Verification items for the finished model (mm, model axes). Face numbers are marked on the shaded views. A direction names the side the tool comes from. Coordinates: 2 decimals unless noted, no trailing zeros. Order: outer loops, then holes, each group sorted by start corner. A loop starts at its lowest first (then second) coordinate and runs counter-clockwise, first axis right, second up. Notation, with made-up numbers: (88, 8) - (99, 8) arc R17 cw to (99, 37) - close; hole circle Ø11 at (31, 84). An arc over 180 degrees is marked (long way). Answer as CSV lines item,"result". Start each with the question number.
1. Go/stop test with flat-tipped pins: pin 1 (1.5 mm diameter, centred on y = 45.5, z = 10, fed in from -X); pin 2 (4 mm diameter, centred on y = 118, z = -8, fed in from -X); pin 3 (8 mm diameter, centred on x = -62, y = -13, fed in from +Z); pin 4 (8 mm diameter, centred on x = -92, z = -17, fed in from +Y). Record where each tip stops, or that it passes through.
2. Section check A-A (z = 4). Record the cut outline in (x, y).
3. Section check D-D (y = 135). Record the cut outline in (x, z), and give its area (3 significant figures).
4. Section check C-C (x = 0). Record the cut outline in (y, z), and give its area (3 significant figures).
5. Set-up check for the marked faces 1, 2 and 3: record each of +Z, -Z, +X, -X, +Y, -Y from which the full face is reachable in a straight line by a thin tool's end or side.
6. Section check B-B (y = -63.5). Record the cut outline in (x, z), and give its area (3 significant figures).
7. Material ranges on L1, parallel to X at y = -41.5, z = 2; L2, parallel to X at y = -66, z = -9.5; L3, parallel to Z at x = 100, y = -31.5, recorded low to high. Write a range as [from, to].
8. Mould release check, pull along X, two halves, no side actions. Record for the marked faces 4, 5 and 6: pulls with the +X half, pulls with the -X half, needs draft (parallel to the pull), parting line crosses it, or undercut.
from build123d import *

# Parameters (mm, degrees)
SKETCH1_R           = 50
BOSS_EXTRUDE1_DEPTH = 25
BOSS_EXTRUDE2_DEPTH = 10
SKETCH3_R           = 5
BOSS_EXTRUDE3_DEPTH = 1


with BuildPart() as part:
    # Sketch1 → Boss-Extrude1 (new body, symmetric)
    with BuildSketch(Plane.XY):
        Circle(SKETCH1_R)
    extrude(amount=BOSS_EXTRUDE1_DEPTH, both=True)

    # Sketch2 → Boss-Extrude2 (add, symmetric)
    with BuildSketch(Plane.XY):
        with BuildLine():
            Line((-21.510823847, 45.13628759), (-38.875641614, 143.617062891))
            ThreePointArc((-38.875641614, 143.617062891), (0, 153.617062891), (38.875641614, 143.617062891))
            Line((38.875641614, 143.617062891), (21.510823847, 45.13628759))
            ThreePointArc((21.510823847, 45.13628759), (0, 50), (-21.510823847, 45.13628759))
        make_face()
        with BuildLine():
            Line((104.938204074, -105.475824672), (28.333759762, -41.197063703))
            ThreePointArc((28.333759762, -41.197063703), (43.301270189, -25), (49.844583609, -3.939223887))
            Line((49.844583609, -3.939223887), (143.813845688, -38.14123822))
            ThreePointArc((143.813845688, -38.14123822), (133.036278919, -76.808531446), (104.938204074, -105.475824672))
        make_face()
        with BuildLine():
            Line((-143.813845688, -38.14123822), (-49.844583609, -3.939223887))
            ThreePointArc((-49.844583609, -3.939223887), (-43.301270189, -25), (-28.333759762, -41.197063703))
            Line((-28.333759762, -41.197063703), (-104.938204074, -105.475824672))
            ThreePointArc((-104.938204074, -105.475824672), (-133.036278919, -76.808531446), (-143.813845688, -38.14123822))
        make_face()
    extrude(amount=BOSS_EXTRUDE2_DEPTH, both=True)

    # Sketch3 → Boss-Extrude3 (add, symmetric)
    with BuildSketch(Plane.XY.offset(10)):
        with Locations((0, 135)):
            Circle(SKETCH3_R)
    extrude(amount=BOSS_EXTRUDE3_DEPTH, both=True)


solid = part.part
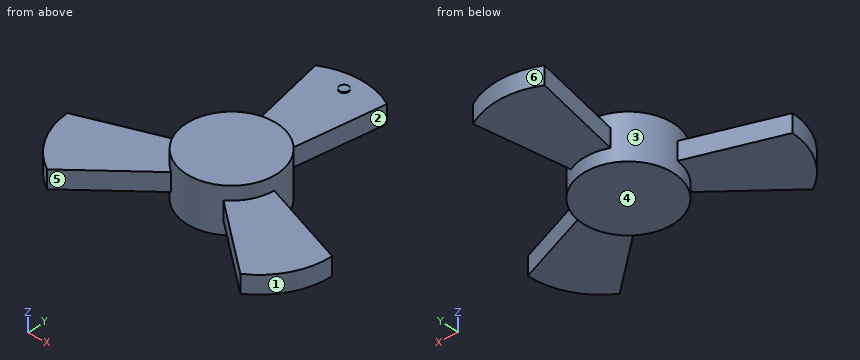
Evaluation:
1,pin 1,"stops at x = -22.3"
1,pin 2,"stops at x = -34.71"
1,pin 3,"stops at z = 10"
1,pin 4,"passes through"
2,outline,"(-143.81, -38.14) arc R80.57 ccw to (-104.94, -105.48) - (-28.33, -41.2) arc R50 ccw to (28.33, -41.2) - (104.94, -105.48) arc R80.57 ccw to (143.81, -38.14) - (49.84, -3.94) arc R50 ccw to (21.51, 45.14) - (38.88, 143.62) arc R80.57 ccw to (-38.88, 143.62) - (-21.51, 45.14) arc R50 ccw to (-49.84, -3.94) - close"
3,outline,"(-37.36, -10) - (37.36, -10) - (37.36, 10) - (5, 10) - (5, 11) - (-5, 11) - (-5, 10) - (-37.36, 10) - close"
3,area,"1,500 mm²"
4,outline,"(-50, -25) - (50, -25) - (50, -10) - (153.62, -10) - (153.62, 10) - (140, 10) - (140, 11) - (130, 11) - (130, 10) - (50, 10) - (50, 25) - (-50, 25) - close"
4,area,"7,080 mm²"
5,face 1,"+Z, -Z, +X, -Y"
5,face 2,"+Z, -Z, +X"
5,face 3,"none"
6,outline,"(-139.18, -10) - (-54.91, -10) - (-54.91, 10) - (-139.18, 10) - close; (54.91, -10) - (139.18, -10) - (139.18, 10) - (54.91, 10) - close"
6,area,"3,370 mm²"
7,L1,"x = [-143.68, -28.69], [-27.89, 27.89], [28.69, 143.68]"
7,L2,"x = [-138.24, -57.89], [57.89, 138.24]"
7,L3,"z = [-10, 10]"
8,face 4,"needs draft"
8,face 5,"undercut"
8,face 6,"parting line crosses it"
